For this review, use the dimensioned drawing (mm, ordinates from the lowest corner) and the shaded views. A direction names the side the tool comes from. Round coordinates to 2 decimals unless told otherwise and drop trailing zeros. Loops run counter-clockwise (first coordinate to the right, second up) from the corner with the lowest first, then second, coordinate; pieces in that order, holes last. Notation, with made-up numbers: (27, 44.25) -> (69, 44.25) arc R30 ccw to (69, 81.25) -> close; hole circle Ø9 at (54, 49). An arc over 180 degrees is marked (long way). Write each question's results on one line, items separated by ' | '.
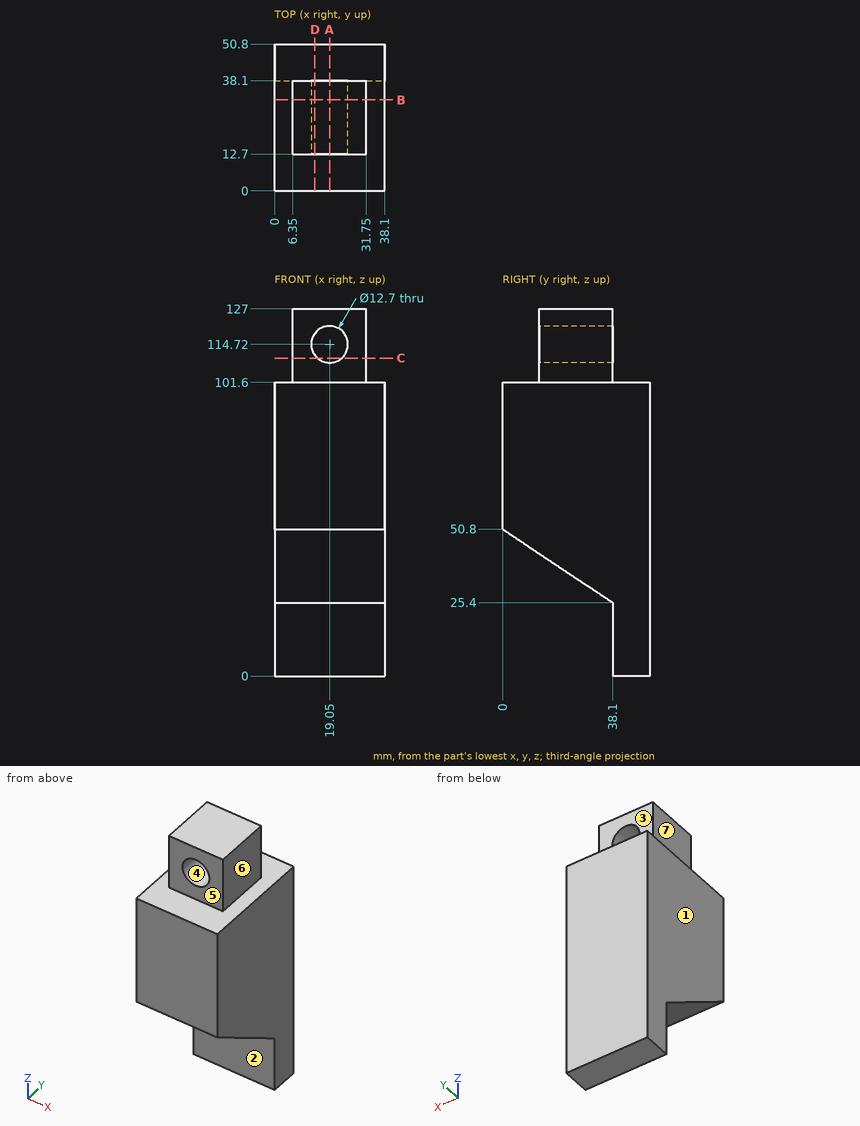
1. Consider section A-A (x = 19.05). State the section outline as (y, z) points.
Values found:
outline: (0, 50.8) -> (38.1, 25.4) -> (38.1, 0) -> (50.8, 0) -> (50.8, 101.6) -> (38.1, 101.6) -> (38.1, 108.37) -> (12.7, 108.37) -> (12.7, 101.6) -> (0, 101.6) -> close; (12.7, 121.07) -> (38.1, 121.07) -> (38.1, 127) -> (12.7, 127) -> close
2. Consider section D-D (x = 14). State the section outline as (y, z) points, plus the area to 3 significant figures.
Values found:
outline: (0, 50.8) -> (38.1, 25.4) -> (38.1, 0) -> (50.8, 0) -> (50.8, 101.6) -> (38.1, 101.6) -> (38.1, 110.87) -> (12.7, 110.87) -> (12.7, 101.6) -> (0, 101.6) -> close; (12.7, 118.57) -> (38.1, 118.57) -> (38.1, 127) -> (12.7, 127) -> close | area: 4,160 mm2
3. To check wall thickness, follow probe 1 along Y at (x, z) = (18, 8); probe 2 along Z at (x, y) = (19.05, 21); probe 3 along Y at (x, z) = (12, 113). State the ranges of each line that lie inside material, in increasing order.
Values found:
probe 1: y = 38.1 to 50.8 | probe 2: z = 36.8 to 108.37, 121.07 to 127 | probe 3: y = 12.7 to 38.1
4. Consider section B-B (y = 31.5). State the section outline as (x, z) points.
Values found:
outline: (0, 29.8) -> (38.1, 29.8) -> (38.1, 101.6) -> (31.75, 101.6) -> (31.75, 127) -> (6.35, 127) -> (6.35, 101.6) -> (0, 101.6) -> close; hole circle Ø12.7 at (19.05, 114.72)
5. For pin 1 (5 mm diameter, centred on x = 30, z = 96, fed in from -Y); pin 2 (20.5 mm diameter, centred on x = 18, z = 120, fed in from -Y); pin 3 (20.5 mm diameter, centred on y = 30.5, z = 113, fed in from -X); pin 4 (8 mm diameter, centred on x = 15, y = 13.5, fed in from -Z), all flat-tipped, find the tip position at first contact; note any pin that passes through.
Values found:
pin 1: stops at y = 0 | pin 2: stops at y = 12.7 | pin 3: stops at x = 6.35 | pin 4: stops at z = 39.13
6. Consider section C-C (z = 110). State the section outline as (x, y) points.
Values found:
outline: (6.35, 12.7) -> (14.8, 12.7) -> (14.8, 38.1) -> (6.35, 38.1) -> close; (23.3, 12.7) -> (31.75, 12.7) -> (31.75, 38.1) -> (23.3, 38.1) -> close
7. Draft analysis for pull direction X (two halves, no side actions). For the marked faces 4, 5, 6 and 7, state which applies: released by +X, released by -X, zero draft, split by the parting line, or undercut.
Values found:
face 4: undercut | face 5: zero draft | face 6: released by +X | face 7: released by -X
8. Tool access review of the marked faces 1, 2 and 3: name each direction out of +Z, -Z, +X, -X, +Y, -Y from which nothing blocks a thin tool from reaching the whole face with its end or side.
Values found:
face 1: +Z, -Z, -X, +Y, -Y | face 2: -Z, +X, -X, -Y | face 3: +Z, +X, -X, +Y
